Input: part model. Units: mm. Frame: model coordinates. Face numbers are marked on the shaded views. Round coordinates to 2 decimals unless told otherwise and drop trailing zeros. Loops run counter-clockwise (first coordinate to the right, second up) from the corner with the lowest first, then second, coordinate; pieces in that order, holes last. Notation, with made-up numbers: (43.25, -10) - (99.25, -10) arc R10 ccw to (99.25, -3) - close; hole circle Ø3 at (36.25, 55.25). An arc over 180 degrees is marked (long way). Use CSV: the item, a comma, the result in double quotes. Start each with the question number.
1. Pin query (flat end, axial travel): P1, Ø1, axis at y = 68.5, z = -74.5, coming from the +X side; P2, Ø0.9, axis at x = 24, z = 6.5, coming from the +Y side; P3, Ø8, axis at x = 54.5, y = 91.5, coming from the +Z side. Return the tip coordinate at first contact, or that it passes through.
2. Cut plane D-D (z = 53.5). Return loops of the section in (x, y), and give its area (3 significant figures).
3. Cut plane C-C (x = 0). Return loops of the section in (y, z), and give its area (3 significant figures).
4. Cut plane B-B (z = 0). Return loops of the section in (x, y), and give its area (3 significant figures).
5. Pull-direction query (X, two-part tool) for the marked faces 1, 2 and 3; classes: +X half, -X half, draft (parallel to the pull), parting line (faces both ways), or undercut.
6. Material intervals for probe 1 along X at (y, z) = (64.5, 0.5); probe 2 along Y at (x, z) = (-26, 6); probe 3 along X at (y, z) = (134, 49.5), sorted ascending. Write a range as from..to.
7. Cut plane A-A (y = 26). Return loops of the section in (x, z), and give its area (3 significant figures).
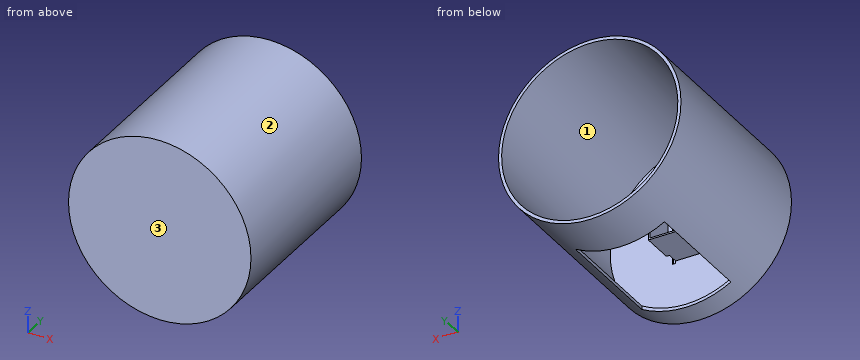
```python
from build123d import *

# Parameters (mm, degrees)
SKETCH_1_R          = 85
EXTRUDE_1_DEPTH     = 180
SHELL_1_T           = 3
SKETCH_2_W          = 86
SKETCH_2_H          = 110
CUT_EXTRUDE_1_DEPTH = 180
SKETCH_3_W          = 47
SKETCH_3_H          = 47
EXTRUDE_2_DEPTH     = 40
SKETCH_4_W          = 55.017876713
SKETCH_4_H          = 12
CUT_EXTRUDE_3_DEPTH = 3


with BuildPart() as part:
    # 草图1 → 凸台-拉伸1 (new body)
    with BuildSketch(Plane(origin=(0, 0, 0), x_dir=(1, 0, 0), z_dir=(0, 1, 0))):
        with Locations(Location((0, 0, 0), (0, 0, 90))):
            Circle(SKETCH_1_R)
    extrude(amount=EXTRUDE_1_DEPTH)

    # 抽壳1
    shell_1_openings = [part.faces().sort_by_distance(p)[0] for p in [
        (0, 180, 0),
    ]]
    offset(amount=SHELL_1_T, openings=shell_1_openings, kind=Kind.INTERSECTION)

    # 草图2 → 切除-拉伸1 (cut)
    with BuildSketch(Plane.XY):
        with Locations((0, 75)):
            Rectangle(SKETCH_2_W, SKETCH_2_H)
    extrude(amount=-CUT_EXTRUDE_1_DEPTH, mode=Mode.SUBTRACT)

    # 草图3 → 凸台-拉伸2 (add)
    with BuildSketch(Plane(origin=(0, 0, 0), x_dir=(1, 0, 0), z_dir=(0, 1, 0))):
        Polygon((0, 25), (25, 25), (25, -25), (-25, -25), (-25, 25), align=None)
        Rectangle(SKETCH_3_W, SKETCH_3_H, mode=Mode.SUBTRACT)
    extrude(amount=EXTRUDE_2_DEPTH)

    # 草图4 → 切除-拉伸3 (cut)
    with BuildSketch(Plane(origin=(25, 0, 0), x_dir=(0, 0, -1), z_dir=(1, 0, 0))):
        with Locations((-0.083732348, 4.206538913)):
            Rectangle(SKETCH_4_W, SKETCH_4_H)
    extrude(amount=-CUT_EXTRUDE_3_DEPTH, mode=Mode.SUBTRACT)


solid = part.part
```
Established:
1,P1,"stops at x = 47.62"
1,P2,"stops at y = 40"
1,P3,"stops at z = 72.07"
2,outline,"(-69.87, -3) - (69.87, -3) - (69.87, 180) - (66.05, 180) - (66.05, 0) - (-66.05, 0) - (-66.05, 180) - (-69.87, 180) - close"
2,area,"1,790 mm2"
3,outline,"(-3, -88) - (20, -88) - (20, -85) - (0, -85) - (0, -25) - (40, -25) - (40, -23.5) - (0, -23.5) - (0, 23.5) - (40, 23.5) - (40, 25) - (0, 25) - (0, 85) - (180, 85) - (180, 88) - (-3, 88) - close; (130, -88) - (180, -88) - (180, -85) - (130, -85) - close"
3,area,"1,400 mm2"
4,outline,"(-88, -3) - (88, -3) - (88, 180) - (85, 180) - (85, 0) - (25, 0) - (25, -1.79) - (22, -1.79) - (22, 0) - (-23.5, 0) - (-23.5, 40) - (-25, 40) - (-25, 0) - (-85, 0) - (-85, 180) - (-88, 180) - close; (23.5, 10.21) - (25, 10.21) - (25, 40) - (23.5, 40) - close"
4,area,"1,710 mm2"
5,face 1,"undercut"
5,face 2,"parting line"
5,face 3,"draft"
6,probe 1,"x = -88..-85, 85..88"
6,probe 2,"y = -3..0"
6,probe 3,"x = -72.76..-69.1, 69.1..72.76"
7,outline,"(-43, -76.78) - (-43, -73.32) arc R85 cw (long way) to (43, -73.32) - (43, -76.78) arc R88 ccw (long way) to start; (-25, -25) - (25, -25) - (25, 25) - (-25, 25) - close; hole (-23.5, -23.5) - (23.5, -23.5) - (23.5, 23.5) - (-23.5, 23.5) - close"
7,area,"1,650 mm2"
